Input: dimensioned drawing with shaded views. Units: mm. Origin: part minimum x, y, z. A direction names the side the tool comes from. Give positions to 0.01 mm unless a question says otherwise; leave off trailing zeros. Loops run counter-clockwise (first coordinate to the right, second up) from the corner with the lowest first, then second, coordinate; pieces in that order, holes last. Notation, with made-up numbers: (82, 86.5) -> (127, 86.5) arc R24 cw to (127, 118.5) -> close; hole circle Ø8 at (66, -7). An arc over 180 degrees is marked (long way). Answer in a Markdown table with one row per item. Add a question column.
1) Line query: line 1 (X direction, y = 3.5, z = 14.5); line 2 (Z direction, x = 7.3, y = 6); line 3 (Z direction, x = 42.5, y = 5.75). Output: solid intervals per line, ascending. Write a range as from..to.
2) Access query for the marked faces 5, 6 and 7. Directions: +Z, -Z, +X, -X, +Y, -Y. A direction counts if a zero-diameter tool reaches every point of the face in a straight line with its end or side. Return the directions, or none.
3) Section query A-A (y = 6). Return the cut outline in (x, z).
4) Section query B-B (z = 13). Return the cut outline in (x, y).
5) First-contact query: P1, Ø3, axis at x = 38.5, y = 4.5, coming from the -Z side; P2, Ø3.5, axis at y = 5.5, z = 10, coming from the +X side; P3, Ø3, axis at x = 2, y = 4, coming from the +Z side; P4, Ø3.5, axis at y = 4.5, z = 8, coming from the -X side. Flat tips, straight axial feed; report the tip coordinate or a pass-through.
6) Section query D-D (y = 11). Return the cut outline in (x, z).
7) Section query C-C (z = 5). Return the cut outline in (x, y).
8) Draft query along Y for the marked faces 1, 2, 3 and 4. Return one class per face: +Y half, -Y half, draft (parallel to the pull), parting line (faces both ways), or undercut.
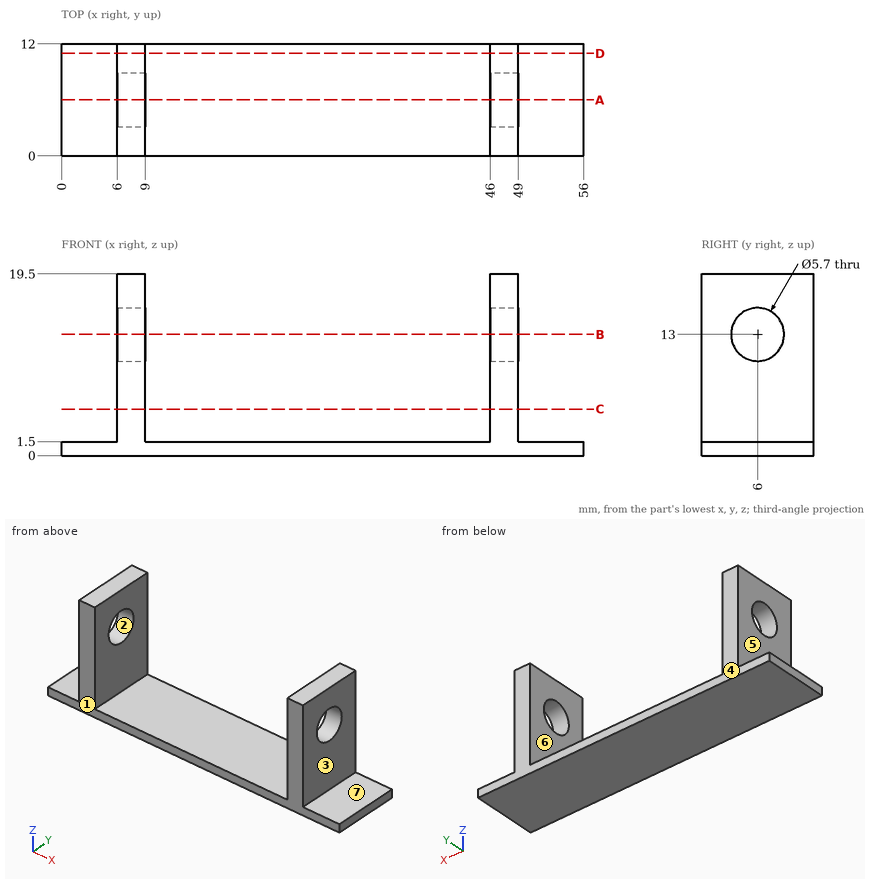
Evaluation:
| question | item | result |
|---|---|---|
| 1 | line 1 | 6..9, 46..49 |
| 1 | line 2 | 0..10.15, 15.85..19.5 |
| 1 | line 3 | 0..1.5 |
| 2 | face 5 | +Z, -X, +Y, -Y |
| 2 | face 6 | +Z, +Y, -Y |
| 2 | face 7 | +Z, +X, +Y, -Y |
| 3 | outline | (0, 0) -> (56, 0) -> (56, 1.5) -> (49, 1.5) -> (49, 10.15) -> (46, 10.15) -> (46, 1.5) -> (9, 1.5) -> (9, 10.15) -> (6, 10.15) -> (6, 1.5) -> (0, 1.5) -> close; (6, 15.85) -> (9, 15.85) -> (9, 19.5) -> (6, 19.5) -> close; (46, 15.85) -> (49, 15.85) -> (49, 19.5) -> (46, 19.5) -> close |
| 4 | outline | (6, 0) -> (9, 0) -> (9, 3.15) -> (6, 3.15) -> close; (6, 8.85) -> (9, 8.85) -> (9, 12) -> (6, 12) -> close; (46, 0) -> (49, 0) -> (49, 3.15) -> (46, 3.15) -> close; (46, 8.85) -> (49, 8.85) -> (49, 12) -> (46, 12) -> close |
| 5 | P1 | z = 0 |
| 5 | P2 | x = 49 |
| 5 | P3 | z = 1.5 |
| 5 | P4 | x = 6 |
| 6 | outline | (0, 0) -> (56, 0) -> (56, 1.5) -> (49, 1.5) -> (49, 19.5) -> (46, 19.5) -> (46, 1.5) -> (9, 1.5) -> (9, 19.5) -> (6, 19.5) -> (6, 1.5) -> (0, 1.5) -> close |
| 7 | outline | (6, 0) -> (9, 0) -> (9, 12) -> (6, 12) -> close; (46, 0) -> (49, 0) -> (49, 12) -> (46, 12) -> close |
| 8 | face 1 | -Y half |
| 8 | face 2 | undercut |
| 8 | face 3 | draft |
| 8 | face 4 | +Y half |
